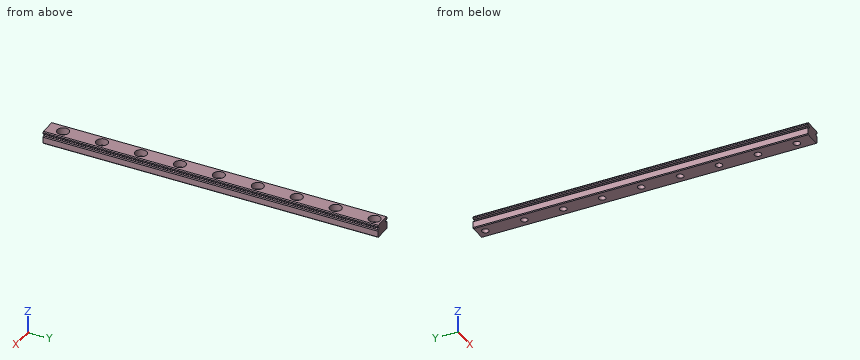
from build123d import *

# Parameters (mm, degrees)
RESSALTO_EXTRUS_O1_DEPTH                             = 1000
CORTE_EXTRUS_O1_START                                = -1000
CORTE_EXTRUS_O1_DEPTH                                = 1000
CORTE_EXTRUS_O2_DEPTH                                = 1001.031261626
CORTE_EXTRUS_O3_DEPTH                                = 1001.031261626
CORTE_EXTRUS_O4_DEPTH                                = 1001.031261626
CORTE_EXTRUS_O5_DEPTH                                = 0.002166667
CORTE_EXTRUS_O6_DEPTH                                = 0.002166667
CORTE_EXTRUS_O7_DEPTH                                = 0.002166667
CORTE_EXTRUS_O8_DEPTH                                = 0.002166667
INCLINA_O1_ANGLE                                     = 45.1469538
ESBO_O10_W                                           = 0.450000001
ESBO_O10_H                                           = 1000
REBAIXO_PARA_PARAFUSO_DE_M_QUINA_DE_CABE_D           = 3.5
REBAIXO_PARA_PARAFUSO_DE_M_QUINA_DE_CABE_CBORE_D     = 6
REBAIXO_PARA_PARAFUSO_DE_M_QUINA_DE_CABE_CBORE_DEPTH = 3.50000002
CHANFRO1_SIZE                                        = 0.062563219
CHANFRO1_SIZE2                                       = 0.062205617
CHANFRO3_START                                       = -3.730761794
CHANFRO3_DEPTH                                       = 0.399013115
CHANFRO4_SIZE                                        = 0.4
FILETE1_R                                            = 0.130000023
SKETCH1_W                                            = 36.072768502
SKETCH1_H                                            = 659.552877555
SKETCH1_W_2                                          = 21.632087489
SKETCH1_H_2                                          = 215.829832124
CUT_EXTRUDE1_DEPTH                                   = 10


with BuildPart() as part:
    # Esboço1 → Ressalto-extrusão1 (new body)
    with BuildSketch(Plane.XZ):
        with BuildLine():
            Line((4.5, 5.4097155), (4.5, 6.01167813))
            Line((4.5, 6.01167813), (4.1, 6.50000002))
            Line((4.1, 6.50000002), (-4.1, 6.50000002))
            Line((-4.1, 6.50000002), (-4.5, 6.01167813))
            Line((-4.5, 6.01167813), (-4.5, 2e-08))
            Line((-4.5, 2e-08), (4.5, 2e-08))
            Line((4.5, 2e-08), (4.5, 3.50196265))
            ThreePointArc((4.5, 3.50196265), (4.477413879, 3.553810372), (4.43494978, 3.59116167))
            ThreePointArc((4.43494978, 3.59116167), (3.930462682, 4.43021964), (4.43494978, 5.26927761))
            ThreePointArc((4.43494978, 5.26927761), (4.490651601, 5.328761203), (4.5, 5.4097155))
        make_face()
    extrude(amount=-RESSALTO_EXTRUS_O1_DEPTH)

    # Esboço2 → Corte-extrusão1 (cut)
    with BuildSketch(Plane(origin=(0, 1000, 0), x_dir=(-1, 0, 0), z_dir=(0, 1, 0)).offset(CORTE_EXTRUS_O1_START)):
        with BuildLine():
            Line((-4.030498711, 4.00588336), (-3.673447948, 4.00588336))
            ThreePointArc((-3.673447948, 4.00588336), (-3.223447946, 4.455883362), (-3.673447948, 4.905883363))
            Line((-3.673447948, 4.905883363), (-3.953580008, 4.905883363))
            ThreePointArc((-3.953580008, 4.905883363), (-4.010719931, 4.899199784), (-4.065149208, 4.917830263))
            ThreePointArc((-4.065149208, 4.917830263), (-3.93114763, 4.466290066), (-4.030498711, 4.00588336))
        make_face()
    extrude(amount=CORTE_EXTRUS_O1_DEPTH, mode=Mode.SUBTRACT)

    # Esboço3 → Corte-extrusão2 (cut, through all)
    with BuildSketch(Plane(origin=(0, 1000, 0), x_dir=(-1, 0, 0), z_dir=(0, 1, 0))):
        with BuildLine():
            Line((4.5, 4.03150278), (4.5, 4.88017535))
            Line((4.5, 4.88017535), (3.66946318, 4.88017535))
            ThreePointArc((3.66946318, 4.88017535), (3.969667593, 4.455839065), (3.66946318, 4.03150278))
            Line((3.66946318, 4.03150278), (4.5, 4.03150278))
        make_face()
    extrude(amount=-CORTE_EXTRUS_O2_DEPTH, mode=Mode.SUBTRACT)

    # Esboço4 → Corte-extrusão3 (cut, through all)
    with BuildSketch(Plane(origin=(0, 1000, 0), x_dir=(-1, 0, 0), z_dir=(0, 1, 0))):
        with BuildLine():
            Line((4.026513974, 4.88017535), (4.5, 4.88017535))
            Line((4.5, 4.88017535), (4.5, 5.328056964))
            ThreePointArc((4.5, 5.328056964), (4.223646078, 5.145991535), (4.026513974, 4.88017535))
        make_face()
    extrude(amount=-CORTE_EXTRUS_O3_DEPTH, mode=Mode.SUBTRACT)

    # Esboço5 → Corte-extrusão4 (cut, through all)
    with BuildSketch(Plane(origin=(0, 1000, 0), x_dir=(-1, 0, 0), z_dir=(0, 1, 0))):
        with BuildLine():
            Line((4.5, 3.583620931), (4.5, 4.03150278))
            Line((4.5, 4.03150278), (4.026513856, 4.03150278))
            ThreePointArc((4.026513856, 4.03150278), (4.223645982, 3.76568645), (4.5, 3.583620931))
        make_face()
    extrude(amount=-CORTE_EXTRUS_O4_DEPTH, mode=Mode.SUBTRACT)

    # Esboço6 → Corte-extrusão5 (cut)
    with BuildSketch(Plane(origin=(0, 1000, 0), x_dir=(-1, 0, 0), z_dir=(0, 1, 0))):
        Polygon((0.891369267, 3.403698133), (0.714701433, 3.168235633), (0.2187042, 2.61105), (1.0945792, 2.61105), (1.0945792, 2.695983333), (0.398689633, 2.695983333), (0.794326433, 3.149466667), (0.9743123, 3.3891), (1.067110588, 3.573407857), (0.95413722, 3.802321701), (0.7876908, 3.88505), (0.54301, 3.88505), (0.375434678, 3.803592619), (0.295011167, 3.6384023), (0.295011167, 3.562), (0.3812718, 3.562), (0.3812718, 3.631766667), (0.437672733, 3.743620833), (0.549645633, 3.800116667), (0.7802262, 3.800116667), (0.893028067, 3.743810633), (0.976240026, 3.576039029), align=None)
    extrude(amount=-CORTE_EXTRUS_O5_DEPTH, mode=Mode.SUBTRACT)

    # Esboço7 → Corte-extrusão6 (cut)
    with BuildSketch(Plane.XZ):
        Polygon((-0.214632167, 3.88505), (-0.953983333, 3.88505), (-0.953983333, 2.61105), (-0.214632167, 2.61105), (-0.214632167, 2.695983333), (-0.86905, 2.695983333), (-0.86905, 3.205583333), (-0.5123963, 3.205583333), (-0.5123963, 3.290516667), (-0.86905, 3.290516667), (-0.86905, 3.800116667), (-0.214632167, 3.800116667), align=None)
    extrude(amount=-CORTE_EXTRUS_O6_DEPTH, mode=Mode.SUBTRACT)

    # Esboço8 → Corte-extrusão7 (cut)
    with BuildSketch(Plane(origin=(0, 1000, 0), x_dir=(-1, 0, 0), z_dir=(0, 1, 0))):
        Polygon((-0.214632167, 3.88505), (-0.953983333, 3.88505), (-0.953983333, 2.61105), (-0.214632167, 2.61105), (-0.214632167, 2.695983333), (-0.86905, 2.695983333), (-0.86905, 3.205583333), (-0.5123963, 3.205583333), (-0.5123963, 3.290516667), (-0.86905, 3.290516667), (-0.86905, 3.800116667), (-0.214632167, 3.800116667), align=None)
    extrude(amount=-CORTE_EXTRUS_O7_DEPTH, mode=Mode.SUBTRACT)

    # Esboço9 → Corte-extrusão8 (cut)
    with BuildSketch(Plane.XZ):
        Polygon((0.510057167, 3.620830633), (0.6071, 3.718655633), (0.6071, 2.609403333), (0.692033333, 2.609403333), (0.692033333, 3.883403333), (0.6741176, 3.883403333), (0.6741176, 3.795069794), (0.3690544, 3.640736667), (0.3690544, 3.551253333), align=None)
    extrude(amount=-CORTE_EXTRUS_O8_DEPTH, mode=Mode.SUBTRACT)

    # Inclinação1
    inclina_o1_faces = [part.faces().sort_by_distance(p)[0] for p in [
        (0.6741176, 0.001083333, 3.839236564),
    ]]
    draft(inclina_o1_faces, Plane(origin=(0.692033333, 0.002166667, 3.883403333), x_dir=(-1, 0, 0), z_dir=(0, 0, -1)), INCLINA_O1_ANGLE)

    # Esboço10 → Corte-Revolução1 (revolve, cut)
    with BuildSketch(Plane.XY.offset(4.455839065)):
        with Locations((-3.294667591, 500)):
            Rectangle(ESBO_O10_W, ESBO_O10_H)
    revolve(axis=Axis((-3.519667591, 1000, 4.455839065), (0, -1, 0)), mode=Mode.SUBTRACT)

    # Rebaixo para parafuso de máquina de cabeça sextavada de M31 (through all)
    with Locations(Plane.XY.offset(6.50000002)):
        with Locations((0, 990), (0, 970), (0, 950), (0, 930), (0, 910), (0, 890), (0, 870), (0, 850), (0, 830), (0, 810), (0, 790), (0, 770), (0, 750), (0, 730), (0, 710), (0, 690), (0, 670), (0, 650), (0, 630), (0, 610), (0, 590), (0, 570), (0, 550), (0, 530), (0, 510), (0, 490), (0, 470), (0, 450), (0, 430), (0, 410), (0, 390), (0, 370), (0, 350), (0, 330), (0, 310), (0, 290), (0, 270), (0, 250), (0, 230), (0, 210), (0, 190), (0, 170), (0, 150), (0, 130), (0, 110), (0, 90), (0, 70), (0, 50), (0, 30), (0, 10)):
            CounterBoreHole(REBAIXO_PARA_PARAFUSO_DE_M_QUINA_DE_CABE_D / 2, REBAIXO_PARA_PARAFUSO_DE_M_QUINA_DE_CABE_CBORE_D / 2, REBAIXO_PARA_PARAFUSO_DE_M_QUINA_DE_CABE_CBORE_DEPTH)

    # Chanfro1
    chanfro1_edges = [part.edges().sort_by_distance(p)[0] for p in [
        (-0.976240026, 999.998916667, 3.576039029),
    ]]
    chanfro1_side = [part.faces().sort_by_distance(p)[0] for p in [
        (-0.933804646, 999.998916667, 3.489868581),
    ]]
    chamfer(chanfro1_edges, length=CHANFRO1_SIZE, length2=CHANFRO1_SIZE2, reference=chanfro1_side[0])

    # Chanfro3: read off the stored shape, not the designer's step
    # Chanfro3 outline → Chanfro3 (add)
    with BuildSketch(Plane(origin=(0, 0, 0), x_dir=(0.8991051825477068, 0, 0.43773264753254887), z_dir=(0.4377326475325489, 0, -0.8991051825477069)).offset(CHANFRO3_START)):
        Polygon((1.327401403, -999.997833333), (1.31122788, -999.997833333), (1.311999664, -1000), (1.327401403, -1000), align=None)
    extrude(amount=CHANFRO3_DEPTH)

    # Chanfro4
    chanfro4_edges = [part.edges().sort_by_distance(p)[0] for p in [
        (4.5, 500, 2e-08),
        (-4.5, 500, 2e-08),
    ]]
    chamfer(chanfro4_edges, length=CHANFRO4_SIZE)

    # Filete1
    filete1_edges = [part.edges().sort_by_distance(p)[0] for p in [
        (4.030498711, 500, 4.00588336),
        (-4.026513974, 500, 4.88017535),
        (-4.5, 500, 5.328056964),
        (-4.5, 500, 3.583620931),
        (-4.026513856, 500, 4.03150278),
    ]]
    fillet(filete1_edges, radius=FILETE1_R)

    # Sketch1 → Cut-Extrude1 (cut)
    with BuildSketch(Plane(origin=(0, 0, 0), x_dir=(-1, 0, 0), z_dir=(0, 0, -1))):
        with Locations((-9.39117436, 683.776438778)):
            Rectangle(SKETCH1_W, SKETCH1_H)
        with Locations((0.25600221, 74.108809522)):
            Rectangle(SKETCH1_W_2, SKETCH1_H_2)
    extrude(amount=-CUT_EXTRUDE1_DEPTH, mode=Mode.SUBTRACT)


solid = part.part
CAD build for the part. Positions are in the model's coordinates, mm. Round coordinates to 2 decimals unless told otherwise and drop trailing zeros. Write each loop counter-clockwise with the first axis right and the second up, starting at its lowest first coordinate (ties: lowest second). Pieces come first, ordered by that corner, then holes. Notation, with made-up numbers: (27, 36.25) -> (52, 36.25) arc R11 cw to (52, 40.25) -> close; hole circle Ø3 at (69, -13). An arc over 180 degrees is marked (long way). Answer as a JSON object with one key per item and string values.
(1) Probe probe 1 along Z at (x, y) = (4, 254); probe 2 along X at (y, z) = (302.5, 0.75); probe 3 along X at (y, z) = (269, 5.5). List the from-to ranges inside material, lowest first. Write a range as [from, to].
Reported:
{"probe 1": "z = [0, 4], [4.9, 6.5]", "probe 2": "x = [-4.5, 4.5]", "probe 3": "x = [-4.5, -2.83], [2.83, 4.5]"}
(2) Pin check, flat tip, straight feed: P1, Ø3, axis at x = 0.5, y = 250.5, coming from the +Z side. Stop position of the tip, or through.
Reported:
{"P1": "stops at z = 3"}
(3) Band-saw the part on A-A, the plane y = 339. List the corners of the cut face in (x, z).
Reported:
{"outline": "(-4.5, 0.4) -> (-4.1, 0) -> (4.1, 0) -> (4.5, 0.4) -> (4.5, 3.5) arc R0.13 ccw to (4.43, 3.59) arc R0.95 cw to (4.07, 3.94) arc R0.13 ccw to (3.95, 4.01) -> (3.67, 4.01) arc R0.45 cw to (3.67, 4.91) -> (3.95, 4.91) arc R0.13 ccw to (4.07, 4.92) arc R0.95 cw to (4.43, 5.27) arc R0.13 ccw to (4.5, 5.41) -> (4.5, 6.01) -> (4.1, 6.5) -> (-4.1, 6.5) -> (-4.5, 6.01) -> (-4.5, 5.41) arc R0.13 ccw to (-4.43, 5.29) arc R0.95 cw to (-4.06, 4.94) arc R0.13 ccw to (-3.95, 4.88) -> (-3.67, 4.88) arc R0.45 cw (long way) to (-3.67, 4.03) -> (-3.95, 4.03) arc R0.13 ccw to (-4.06, 3.97) arc R0.95 cw to (-4.43, 3.62) arc R0.13 ccw to (-4.5, 3.5) -> close"}
(4) Band-saw the part on B-B, the plane z = 1.75. Count the separate pieces of the cut face and the enclosed holes in it, then the cut area to 3 significant figures.
Reported:
{"separate pieces": "1", "enclosed holes": "9", "area": "1,460 mm^2"}
